from build123d import *

# Parameters (mm, degrees)
F0_W         = 68
F0_H         = 30
F1_DEPTH     = 19.5
F2_R         = 2.5
F3_DEPTH     = 19.5
F4_W         = 10
F4_H         = 13
F4_W_2       = 8
F4_H_2       = 14
F5_DEPTH     = 5
F6_T1_DEPTH  = 20
F6_T3_DEPTH  = 26
F6_T5_DEPTH  = 20
F6_T7_DEPTH  = 12
F6_T9_DEPTH  = 12
F6_T11_DEPTH = 22.5
F6_S15_W     = 2
F6_S15_H     = 2
F6_T16_DEPTH = 2
F6_S21_W     = 2
F6_S21_H     = 2
F6_T22_DEPTH = 2
F6_S27_W     = 2
F6_S27_H     = 2
F6_T28_DEPTH = 2
F6_S33_W     = 2
F6_S33_H     = 2
F6_T34_DEPTH = 2


# Not quite as in the source:
# - a fillet or chamfer that OpenCascade refuses, or shapes differently, is made with other operations: its cross-section is extruded or revolved along the edge and cut away or added


with BuildPart() as f1:
    # F0 (on Top) → F1 (new body)
    with BuildSketch(Plane.XY):
        Rectangle(F0_W, F0_H)
    extrude(amount=F1_DEPTH)

    # F2 (on face) → F3 (cut, through all)
    with BuildSketch(Plane.XY.offset(19.5)):
        with Locations((-28.5, 0)):
            Circle(F2_R)
        with Locations((28.5, 0)):
            Circle(F2_R)
    extrude(amount=-F3_DEPTH, mode=Mode.SUBTRACT)

    # F4 (on face) → F5 (cut)
    with BuildSketch(Plane.XY.offset(19.5)):
        with Locations((0, 8.5)):
            Rectangle(F4_W, F4_H)
        with Locations((12, 8.5)):
            Rectangle(F4_W, F4_H)
        with Locations((-12, 8.5)):
            Rectangle(F4_W, F4_H)
        with Locations((-12, -8.5)):
            Rectangle(F4_W, F4_H)
        with Locations((0, -8.5)):
            Rectangle(F4_W, F4_H)
        with Locations((12, -8.5)):
            Rectangle(F4_W, F4_H)
        with Locations((29, 0)):
            Rectangle(F4_W_2, F4_H_2)
        with Locations((-29, 0)):
            Rectangle(F4_W_2, F4_H_2)
    extrude(amount=-F5_DEPTH, mode=Mode.SUBTRACT)

    # F6: fillet of radius 2 on 14 edges, made by hand

    # F6_s2 → F6_t1 (cut)
    with BuildSketch(Plane.YZ.offset(-32)):
        with BuildLine():
            ThreePointArc((-15, 17.5), (-14.4142135624, 18.9142135624), (-13, 19.5))
            Line((-13, 19.5), (-15, 19.5))
            Line((-15, 19.5), (-15, 17.5))
        make_face()
        with BuildLine():
            ThreePointArc((13, 19.5), (14.4142135624, 18.9142135624), (15, 17.5))
            Line((15, 17.5), (15, 19.5))
            Line((15, 19.5), (13, 19.5))
        make_face()
    extrude(amount=F6_T1_DEPTH, mode=Mode.SUBTRACT)

    # F6_s4 → F6_t3 (cut)
    with BuildSketch(Plane.XZ.offset(-13)):
        with BuildLine():
            ThreePointArc((-32, 19.5), (-33.4142135624, 18.9142135624), (-34, 17.5))
            Line((-34, 17.5), (-34, 19.5))
            Line((-34, 19.5), (-32, 19.5))
        make_face()
        with BuildLine():
            ThreePointArc((34, 17.5), (33.4142135624, 18.9142135624), (32, 19.5))
            Line((32, 19.5), (34, 19.5))
            Line((34, 19.5), (34, 17.5))
        make_face()
    extrude(amount=F6_T3_DEPTH, mode=Mode.SUBTRACT)

    # F6_s6 → F6_t5 (cut)
    with BuildSketch(Plane.YZ.offset(12)):
        with BuildLine():
            ThreePointArc((-15, 17.5), (-14.4142135624, 18.9142135624), (-13, 19.5))
            Line((-13, 19.5), (-15, 19.5))
            Line((-15, 19.5), (-15, 17.5))
        make_face()
        with BuildLine():
            ThreePointArc((13, 19.5), (14.4142135624, 18.9142135624), (15, 17.5))
            Line((15, 17.5), (15, 19.5))
            Line((15, 19.5), (13, 19.5))
        make_face()
    extrude(amount=F6_T5_DEPTH, mode=Mode.SUBTRACT)

    # F6_s8 → F6_t7 (cut)
    with BuildSketch(Plane.YZ):
        with BuildLine():
            ThreePointArc((-15, 17.5), (-14.4142135624, 18.9142135624), (-13, 19.5))
            Line((-13, 19.5), (-15, 19.5))
            Line((-15, 19.5), (-15, 17.5))
        make_face()
        with BuildLine():
            ThreePointArc((13, 19.5), (14.4142135624, 18.9142135624), (15, 17.5))
            Line((15, 17.5), (15, 19.5))
            Line((15, 19.5), (13, 19.5))
        make_face()
    extrude(amount=F6_T7_DEPTH, mode=Mode.SUBTRACT)

    # F6_s10 → F6_t9 (cut)
    with BuildSketch(Plane.YZ.offset(-12)):
        with BuildLine():
            ThreePointArc((-15, 17.5), (-14.4142135624, 18.9142135624), (-13, 19.5))
            Line((-13, 19.5), (-15, 19.5))
            Line((-15, 19.5), (-15, 17.5))
        make_face()
        with BuildLine():
            ThreePointArc((13, 19.5), (14.4142135624, 18.9142135624), (15, 17.5))
            Line((15, 17.5), (15, 19.5))
            Line((15, 19.5), (13, 19.5))
        make_face()
    extrude(amount=F6_T9_DEPTH, mode=Mode.SUBTRACT)

    # F6_s12 → F6_t11 (cut)
    with BuildSketch(Plane.XY.offset(-5)):
        with BuildLine():
            ThreePointArc((-32, -15), (-33.4142135624, -14.4142135624), (-34, -13))
            Line((-34, -13), (-34, -15))
            Line((-34, -15), (-32, -15))
        make_face()
        with BuildLine():
            ThreePointArc((-34, 13), (-33.4142135624, 14.4142135624), (-32, 15))
            Line((-32, 15), (-34, 15))
            Line((-34, 15), (-34, 13))
        make_face()
        with BuildLine():
            ThreePointArc((34, 13), (33.4142135624, 14.4142135624), (32, 15))
            Line((32, 15), (34, 15))
            Line((34, 15), (34, 13))
        make_face()
        with BuildLine():
            ThreePointArc((32, -15), (33.4142135624, -14.4142135624), (34, -13))
            Line((34, -13), (34, -15))
            Line((34, -15), (32, -15))
        make_face()
    extrude(amount=F6_T11_DEPTH, mode=Mode.SUBTRACT)


with BuildPart() as f6_tool14:
    # F6_s15 → F6_t16 (new body)
    with BuildSketch(Plane.XZ.offset(13)):
        with Locations((-33, 18.5)):
            Rectangle(F6_S15_W, F6_S15_H)
    extrude(amount=F6_T16_DEPTH)

    # F6_s17 → F6_t18 (revolve, cut)
    with BuildSketch(Plane(origin=(-32, -13, 17.5), x_dir=(0.7071067812, 0, -0.7071067812), z_dir=(-0.7071067812, 0, -0.7071067812))):
        with BuildLine():
            ThreePointArc((0, -2), (2, 0), (0, 2))
            Line((0, 2), (0, -2))
        make_face()
    revolve(axis=Axis((-32, -13, 17.5), (0, -1, 0)), mode=Mode.SUBTRACT)


with BuildPart() as f1_1:
    add(f1.part)

    # F6_t13: cut F6_tool14
    add(f6_tool14.part, mode=Mode.SUBTRACT)


with BuildPart() as f6_tool20:
    # F6_s21 → F6_t22 (new body)
    with BuildSketch(Plane.XY.offset(17.5)):
        with Locations((-33, 14)):
            Rectangle(F6_S21_W, F6_S21_H)
    extrude(amount=F6_T22_DEPTH)

    # F6_s23 → F6_t24 (revolve, cut)
    with BuildSketch(Plane(origin=(-32, 13, 17.5), x_dir=(0.7071067812, -0.7071067812, 0), z_dir=(-0.7071067812, -0.7071067812, 0))):
        with BuildLine():
            ThreePointArc((0, -2), (2, 0), (0, 2))
            Line((0, 2), (0, -2))
        make_face()
    revolve(axis=Axis((-32, 13, 17.5), (0, 0, 1)), mode=Mode.SUBTRACT)


with BuildPart() as f1_2:
    add(f1_1.part)

    # F6_t19: cut F6_tool20
    add(f6_tool20.part, mode=Mode.SUBTRACT)


with BuildPart() as f6_tool26:
    # F6_s27 → F6_t28 (new body)
    with BuildSketch(Plane.XZ.offset(13)):
        with Locations((33, 18.5)):
            Rectangle(F6_S27_W, F6_S27_H)
    extrude(amount=F6_T28_DEPTH)

    # F6_s29 → F6_t30 (revolve, cut)
    with BuildSketch(Plane(origin=(32, -13, 17.5), x_dir=(-0.7071067812, 0, -0.7071067812), z_dir=(-0.7071067812, 0, 0.7071067812))):
        with BuildLine():
            ThreePointArc((0, -2), (2, 0), (0, 2))
            Line((0, 2), (0, -2))
        make_face()
    revolve(axis=Axis((32, -13, 17.5), (0, -1, 0)), mode=Mode.SUBTRACT)


with BuildPart() as f1_3:
    add(f1_2.part)

    # F6_t25: cut F6_tool26
    add(f6_tool26.part, mode=Mode.SUBTRACT)


with BuildPart() as f6_tool32:
    # F6_s33 → F6_t34 (new body)
    with BuildSketch(Plane.YZ.offset(32)):
        with Locations((14, 18.5)):
            Rectangle(F6_S33_W, F6_S33_H)
    extrude(amount=F6_T34_DEPTH)

    # F6_s35 → F6_t36 (revolve, cut)
    with BuildSketch(Plane(origin=(32, 13, 17.5), x_dir=(0, -0.7071067812, -0.7071067812), z_dir=(0, -0.7071067812, 0.7071067812))):
        with BuildLine():
            ThreePointArc((0, -2), (2, 0), (0, 2))
            Line((0, 2), (0, -2))
        make_face()
    revolve(axis=Axis((32, 13, 17.5), (1, 0, 0)), mode=Mode.SUBTRACT)


with BuildPart() as f1_4:
    add(f1_3.part)

    # F6_t31: cut F6_tool32
    add(f6_tool32.part, mode=Mode.SUBTRACT)


solid = f1_4.part
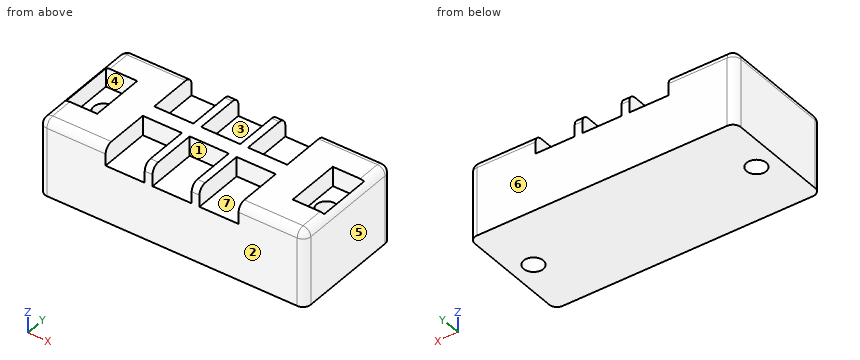
Model file for the job. Use its own axes, mm. Face numbers are marked on the shaded views. A direction names the side the tool comes from. Give positions to 0.01 mm unless a question says otherwise; leave off trailing zeros. Write each loop counter-clockwise with the first axis right and the second up, starting at its lowest first coordinate (ties: lowest second). Pieces come first, ordered by that corner, then holes. Notation, with made-up numbers: (68.5, -25) -> (111.5, -25) arc R4 ccw to (111.5, -20) -> close; hole circle Ø3 at (-20.5, -28). An arc over 180 degrees is marked (long way). Write item = value, one per line.
(1) Slice it at C-C, the plane z = 4.75. Give the cut face in (x, y).
Determined:
outline = (-34, -13) arc R2 ccw to (-32, -15) -> (32, -15) arc R2 ccw to (34, -13) -> (34, 13) arc R2 ccw to (32, 15) -> (-32, 15) arc R2 ccw to (-34, 13) -> close; hole circle Ø5 at (-28.5, 0); hole circle Ø5 at (28.5, 0)
(2) Tool access for the marked faces 1, 2, 3 and 4: list every direction of +Z, -Z, +X, -X, +Y, -Y with a clear straight run to the whole face (end or side of a thin tool).
Determined:
face_1 = +Z, -Y
face_2 = +Z, -Z, +X, -X, -Y
face_3 = +Z, +Y
face_4 = +Z
(3) Probe line 1 along X through (y, z) = (6.5, 16); line 2 along X through (y, z) = (1, 2); line 3 along X through (y, z) = (-1.5, 9). List the from-to ranges inside material, lowest first.
Determined:
line_1 = -34 to -33, -25 to -17, -7 to -5, 5 to 7, 17 to 25, 33 to 34
line_2 = -34 to -30.79, -26.21 to 26.21, 30.79 to 34
line_3 = -34 to -30.5, -26.5 to 26.5, 30.5 to 34
(4) Slice it at A-A, the plane x = 28.5. Give the cut face in (y, z), then the cut area to 3 significant figures.
Determined:
outline = (-15, 0) -> (-2.5, 0) -> (-2.5, 14.5) -> (-7, 14.5) -> (-7, 19.5) -> (-13, 19.5) arc R2 ccw to (-15, 17.5) -> close; (2.5, 0) -> (15, 0) -> (15, 17.5) arc R2 ccw to (13, 19.5) -> (7, 19.5) -> (7, 14.5) -> (2.5, 14.5) -> close
area = 441 mm2
(5) Flat gauge pins, fed straight in: P1, Ø6, axis at x = 28.5, y = 0, coming from the -Z side; P2, Ø6, axis at x = -28.5, y = 0, coming from the +Z side; P3, Ø2.5, axis at x = 14, z = 17.5, coming from the +Y side. Where does each tip first touch, or does it go through?
Determined:
P1 = 0
P2 = 14.5
P3 = 2
(6) Slice it at D-D, the plane x = 2. Give the cut face in (y, z), then the cut area to 3 significant figures.
Determined:
outline = (-15, 0) -> (15, 0) -> (15, 14.5) -> (2, 14.5) -> (2, 19.5) -> (-2, 19.5) -> (-2, 14.5) -> (-15, 14.5) -> close
area = 455 mm2
(7) Mould opens along X. For the marked faces 5, 6 and 7 say: released by +X, released by -X, zero draft, split by the parting line, or undercut.
Determined:
face_5 = released by +X
face_6 = zero draft
face_7 = undercut
(8) Slice it at B-B, the plane y = 0. Give the cut face in (x, z).
Determined:
outline = (-34, 0) -> (-31, 0) -> (-31, 14.5) -> (-33, 14.5) -> (-33, 19.23) arc R2 ccw to (-34, 17.5) -> close; (-26, 0) -> (26, 0) -> (26, 14.5) -> (25, 14.5) -> (25, 19.5) -> (-25, 19.5) -> (-25, 14.5) -> (-26, 14.5) -> close; (31, 0) -> (34, 0) -> (34, 17.5) arc R2 ccw to (33, 19.23) -> (33, 14.5) -> (31, 14.5) -> close
